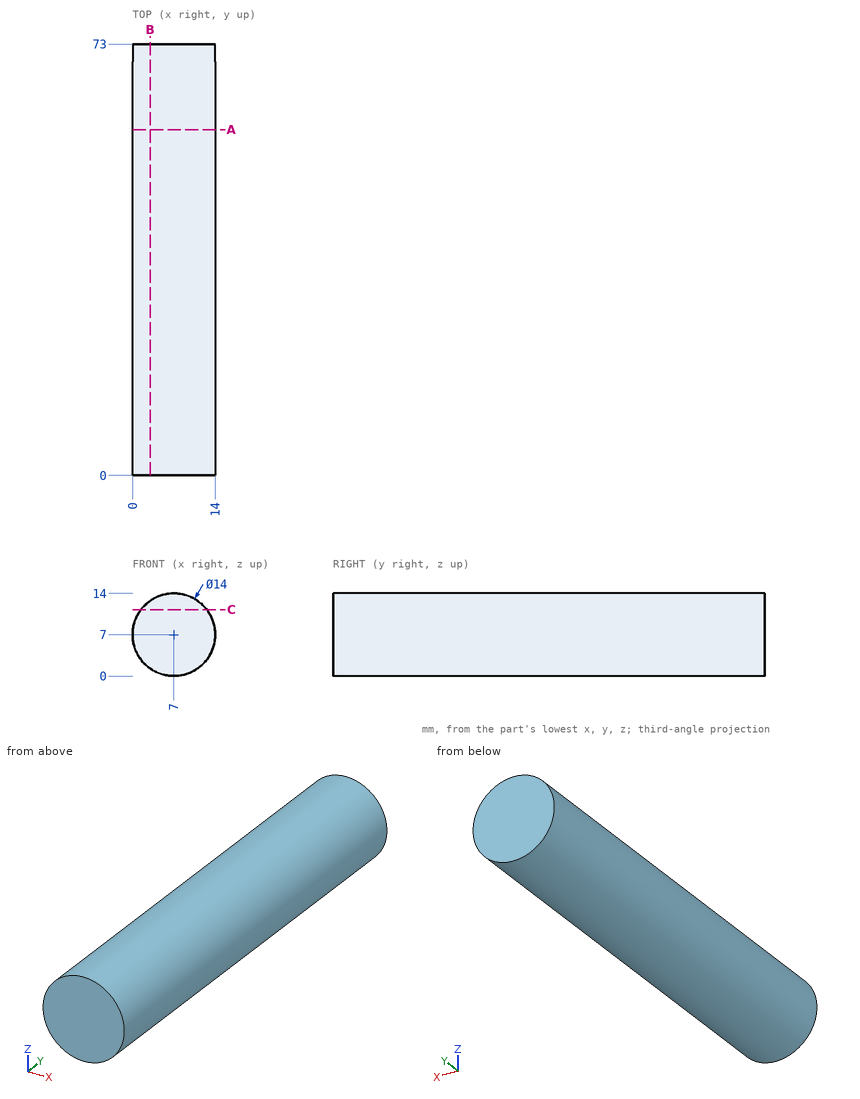
Print and shaded views of the part. All mm, measured from the part's lowest x, y and z. Coordinates: 2 decimals unless noted, no trailing zeros. Loops run counter-clockwise (first coordinate to the right, second up) from the corner with the lowest first, then second, coordinate; pieces in that order, holes last. Notation, with made-up numbers: (-27.5, -27) -> (-2.5, -27) arc R25 ccw to (-2.5, -4) -> close; hole circle Ø7 at (28.5, -27). An arc over 180 degrees is marked (long way). Use one line per item in the form item = value. Start each with the question number.
(1) Probe probe 1 along X at (y, z) = (24, 4.5); probe 2 along X at (y, z) = (23.5, 3.5); probe 3 along Z at (x, y) = (13.25, 27). List the from-to ranges inside material, lowest first. Write a range as from..to.
(2) Cut at B-B on x = 3. Give the cut face in (y, z).
(3) Cut at A-A on y = 58.5. Give the cut face in (x, z), and give its area (3 significant figures).
(4) Cut at C-C on z = 11.25. Give the cut face in (x, y), and give its area (3 significant figures).
(5) Flat gauge pins, fed straight in: pin 1 (6 mm diameter, centred on y = 42.5, z = 2.5, fed in from +X); pin 2 (1 mm diameter, centred on x = 1.5, y = 16.5, fed in from -Z). Where does each tip first touch, or does it go through?
Values:
q1.probe_1 = 0.46..13.54
q1.probe_2 = 0.94..13.06
q1.probe_3 = 3.85..10.15
q2.outline = (0, 1.26) -> (73, 1.26) -> (73, 12.74) -> (0, 12.74) -> close
q3.outline = circle Ø14 at (7, 7)
q3.area = 154 mm2
q4.outline = (1.44, 0) -> (12.56, 0) -> (12.56, 73) -> (1.44, 73) -> close
q4.area = 812 mm2
q5.pin_1 = 13.84
q5.pin_2 = 2.1
